```python
from build123d import *

# Parameters (mm, degrees)
CYLINDER022_R     = 7
CYLINDER022_DEPTH = 64


with BuildPart() as obj1:
    # Cone001 → Cone001 (revolve)
    with BuildSketch(Plane(origin=(-99.5, 36.6, 15.125), x_dir=(0, 0, 1), z_dir=(0, -1, 0))):
        Polygon((0, 0), (2, 0), (7, 10.5), (0, 10.5), align=None)
    revolve(axis=Axis((-99.5, 36.6, 15.125), (-1, 0, 0)))


with BuildPart() as fusion012:
    # Cylinder022 → Cylinder022 (new body)
    with BuildSketch(Plane(origin=(-110, 36.6, 15.125), x_dir=(0, 0, 1), z_dir=(-1, 0, 0))):
        Circle(CYLINDER022_R)
    extrude(amount=CYLINDER022_DEPTH)

    # Fusion012: union obj1
    add(obj1.part)


solid = fusion012.part
```
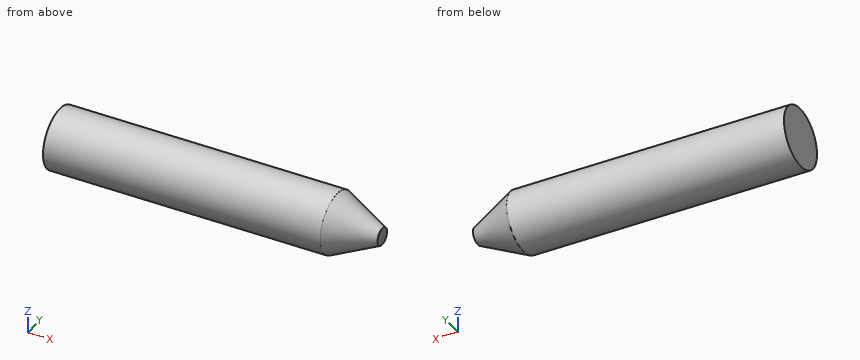
Geometry check sheet. Reference: the model listing, model coordinates, mm. Give positions to 0.01 mm unless a question says otherwise; leave off trailing zeros. Order: outer loops, then holes, each group sorted by start corner. A loop starts at its lowest first (then second) coordinate and runs counter-clockwise, first axis right, second up.
1. Section check A-A, the plane y = 36.6. Enter the section's corners in (x, z) (3 decimals), and give its area (4 significant figures).
2. Section check C-C, the plane x = -107.5. Enter the section's corners in (y, z) (3 decimals), and give its area (3 significant figures).
3. Section check B-B, the plane x = -159. Enter the section's corners in (y, z) (3 decimals), and give its area (3 significant figures).
4. Thickness scan on L1, parallel to Y at x = -126.5, z = 9; L2, parallel to Y at x = -138, z = 14.75; L3, parallel to X at y = 35, z = 17.75. Record the ranges inside material, lowest first.
5. Gauge pin test, flat ends, axial feed: pin 1 Ø1 at (y, z) = (32, 12.5) entering from +X; pin 2 Ø8 at (x, z) = (-119, 20.5) entering from +Y; pin 3 Ø3 at (x, y) = (-110, 32.5) entering from -Z. Record the tip position at first contact, or that the pin passes through.
Values follow:
1. outline: (-174, 8.125) - (-110, 8.125) - (-99.5, 13.125) - (-99.5, 17.125) - (-110, 22.125) - (-174, 22.125) - close
1. area: 990.5 mm2
2. outline: circle Ø11.619 at (36.6, 15.125)
2. area: 106 mm2
3. outline: circle Ø14 at (36.6, 15.125)
3. area: 154 mm2
4. L1: y = 33.21 to 39.99
4. L2: y = 29.61 to 43.59
4. L3: x = -174 to -101.76
5. pin 1: stops at x = -105.37
5. pin 2: stops at y = 43.46
5. pin 3: stops at z = 8.63
